```python
from build123d import *

# Parameters (mm, degrees)
F1_DEPTH = 400
F0_W     = 160
F0_H     = 80
F2_DEPTH = 80
F3_DEPTH = 160
F4_DEPTH = 240
F5_DEPTH = 320
F6_DEPTH = 320
F8_DEPTH = 80


with BuildPart() as f1:
    # F0 (on Top) → F1 (new body)
    with BuildSketch(Plane.XY):
        Polygon((200, 200), (-200, 200), (-200, -200), (-120, -200), (-120, 120), (120, 120), (200, 120), align=None)
    extrude(amount=F1_DEPTH)



with BuildPart() as f2:
    # F0 (on Top) → F2 (new body)
    with BuildSketch(Plane.XY):
        with Locations((40, -160)):
            Rectangle(F0_W, F0_H)
    extrude(amount=F2_DEPTH)

    # F0 (on Top) → F3 (join)
    with BuildSketch(Plane.XY):
        with Locations((40, -80)):
            Rectangle(F0_W, F0_H)
    extrude(amount=F3_DEPTH)

    # F0 (on Top) → F4 (join)
    with BuildSketch(Plane.XY):
        with Locations((40, 0)):
            Rectangle(F0_W, F0_H)
    extrude(amount=F4_DEPTH)


with BuildPart() as f1_1:
    add(f1.part)

    add(f2.part)  # F5 merges F2
    # F0 (on Top) → F5 (join)
    with BuildSketch(Plane.XY):
        Polygon((-120, 120), (-120, -200), (-40, -200), (-40, -120), (-40, -40), (-40, 40), (120, 40), (120, 120), align=None)
    extrude(amount=F5_DEPTH)

    # F0 (on Top) → F6 (join)
    with BuildSketch(Plane.XY):
        Polygon((200, -200), (200, 120), (120, 120), (120, 40), (120, -40), (120, -120), (120, -200), align=None)
    extrude(amount=F6_DEPTH)

    # F7 (on face) → F8 (cut)
    with BuildSketch(Plane.YZ.offset(200)):
        Polygon((-200, 0), (120, 320), (-200, 320), align=None)
    extrude(amount=-F8_DEPTH, mode=Mode.SUBTRACT)


solid = f1_1.part
```
Geometry check sheet. Reference: the model listing, model coordinates, mm. A direction names the side the tool comes from. Coordinates: 2 decimals unless noted, no trailing zeros. Loops run counter-clockwise (first coordinate to the right, second up) from the corner with the lowest first, then second, coordinate; pieces in that order, holes last.
Item 1: Thickness scan on line 1 (Z direction, x = 16, y = -131); line 2 (Y direction, x = 81, z = 166); line 3 (Z direction, x = -46.5, y = -137). Record the ranges inside material, lowest first.
Item 2: Sectioned sample at A-A, the plane z = 119.5. Record the boundary of the cut face in (x, y), then the cut area to 3 significant figures.
Item 3: Access from +Z, -Z, +X, -X, +Y, -Y to the whole of each face (thin tool, end or side, straight path). Record for faces 1 (the face through (39, -40, 199)), 2 (the face through (-3, 3, 0)).
Item 4: Sectioned sample at B-B, the plane y = 13. Record the boundary of the cut face in (x, z).
Item 5: Sectioned sample at C-C, the plane x = 85. Record the boundary of the cut face in (y, z).
Item 6: Go/stop test with flat-tipped pins: pin 1 Ø24 at (x, z) = (63, 295.5) entering from -Y; pin 2 Ø4 at (y, z) = (-152.5, 262.5) entering from +X; pin 3 Ø6 at (x, y) = (-59, -122) entering from +Z. Record where each tip stops, or that it passes through.
Item 7: Sectioned sample at D-D, the plane y = -91.5. Record the boundary of the cut face in (x, z), then the cut area to 3 significant figures.
Check result:
1. line 1: z = 0 to 80
1. line 2: y = -40 to 200
1. line 3: z = 0 to 320
2. outline: (-200, -200) - (-40, -200) - (-40, -120) - (120, -120) - (120, -80.5) - (200, -80.5) - (200, 200) - (-200, 200) - close
2. area: 138,000 mm2
3. face 1: +Z, +X, -Y
3. face 2: -Z, +X, -X, +Y, -Y
4. outline: (-200, 0) - (200, 0) - (200, 213) - (120, 213) - (120, 240) - (-40, 240) - (-40, 320) - (-120, 320) - (-120, 400) - (-200, 400) - close
5. outline: (-200, 0) - (200, 0) - (200, 400) - (120, 400) - (120, 320) - (40, 320) - (40, 240) - (-40, 240) - (-40, 160) - (-120, 160) - (-120, 80) - (-200, 80) - close
6. pin 1: stops at y = 40
6. pin 2: stops at x = -40
6. pin 3: stops at z = 320
7. outline: (-200, 0) - (200, 0) - (200, 108.5) - (120, 108.5) - (120, 160) - (-40, 160) - (-40, 320) - (-120, 320) - (-120, 400) - (-200, 400) - close
7. area: 91,900 mm2
